Part model, mm, in its own coordinate system. Face numbers are marked on the shaded views. A direction names the side the tool comes from. Round coordinates to 2 decimals unless told otherwise and drop trailing zeros. Loops run counter-clockwise (first coordinate to the right, second up) from the corner with the lowest first, then second, coordinate; pieces in that order, holes last. Notation, with made-up numbers: (-32.5, 52.5) -> (-10.5, 52.5) arc R5 cw to (-10.5, 57.5) -> close; hole circle Ø10 at (9.5, -36.5). An arc over 180 degrees is marked (long way). Answer as CSV lines item,"result".
Autodesk Inventor part; units mm, degrees
ref_plane "YZ Plane" through (0, 0, 0) normal (1, 0, 0) x (0, 1, 0)
ref_plane "XZ Plane" through (0, 0, 0) normal (0, 1, 0) x (-1, 0, 0)
ref_plane "XY Plane" through (0, 0, 0) normal (0, 0, 1) x (1, 0, 0)
sketch "Sketch1" plane through (0, 0, 0) normal (0, 1, 0) x (-1, 0, 0)
  circle A0 centre (0, 0) radius 4.953
  circle A1 centre (0, -11.43) radius 4.953
  dimension "d0" = 9.906
  dimension "d1" = 9.906
  dimension "d2" = 11.43
extrude "Extrusion1" add sketch "Sketch1" along normal blind 1.2192
sketch "Sketch2" plane through (0, 1.2192, 0) normal (0, 1, 0) x (1, 0, 0)
  circle A0 centre (0, 0) radius 3.683
  circle A1 centre (0, 11.43) radius 3.683
  dimension "d5" = 7.366
  dimension "d6" = 7.366
  dimension "d7" = 11.43
extrude "Extrusion2" add sketch "Sketch2" along normal blind 6.731
fillet "Fillet1" radius 0.7937 2 edges at (-3.683, 7.9502, -11.43) (-3.683, 7.9502, 0)
sketch "Sketch3" plane through (0, 0, 0) normal (0, -1, 0) x (1, 0, 0)
  circle A0 centre (0, 0) radius 2.8892
  line L0 (-4.953, 0) -> (-6.0325, 0)
  line L1 (-7.62, -1.5875) -> (-7.62, -9.8425)
  line L2 (-4.953, -11.43) -> (-6.0325, -11.43)
  circle A1 centre (0, -11.43) radius 4.953
  line L3 (4.953, -11.4315) -> (6.039, -11.4309)
  line L4 (7.6256, -9.8425) -> (7.6209, -1.5873)
  line L5 (6.0334, -0.0007) -> (4.953, -0.0007)
  line L6 (-6.35, -8.5725) -> (-6.35, -2.8575)
  line L7 (-4.7625, -1.27) -> (-4.7874, -1.27)
  line L8 (-4.7874, -10.16) -> (-4.7625, -10.16)
  circle A2 centre (0, 0) radius 4.953
  line L9 (4.7874, -1.27) -> (4.7641, -1.27)
  line L10 (6.3516, -2.8566) -> (6.3548, -8.5716)
  line L11 (4.7682, -10.16) -> (4.7874, -10.16)
  arc A3 (6.039, -11.4309) -> (7.6256, -9.8425) centre (6.0381, -9.8434) ccw
  arc A4 (4.7682, -10.16) -> (6.3548, -8.5716) centre (4.7673, -8.5725) ccw
  arc A5 (7.6209, -1.5873) -> (6.0334, -0.0007) centre (6.0334, -1.5882) ccw
  arc A6 (6.3516, -2.8566) -> (4.7641, -1.27) centre (4.7641, -2.8575) ccw
  arc A7 (-6.0325, 0) -> (-7.62, -1.5875) centre (-6.0325, -1.5875) ccw
  arc A8 (-4.7625, -1.27) -> (-6.35, -2.8575) centre (-4.7625, -2.8575) ccw
  arc A9 (-6.35, -8.5725) -> (-4.7625, -10.16) centre (-4.7625, -8.5725) ccw
  arc A10 (-7.62, -9.8425) -> (-6.0325, -11.43) centre (-6.0325, -9.8425) ccw
  circle A11 centre (0, -11.43) radius 2.8892
  point P0 (7.6265, -11.43)
  dimension "d12" = 1.27
  dimension "d14" = 1.5875
  dimension "d17" = 7.62
  dimension "d18" = 1.27
  dimension "d21" = 7.62
  dimension "d22" = 1.27
  dimension "d23" = 1.2716
extrude "Extrusion3" add sketch "Sketch3" against normal blind 1.2192 contours A2 A8 L6 A9 A1 L2 A10 L1 A7 L0 | L5 A5 L4 A3 L3 A1 A4 L10 A6 A2
properties part number "push_buttons"
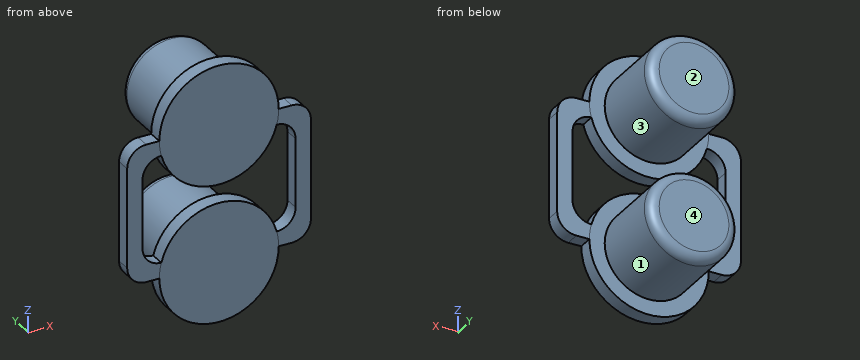
Q1. Saw through at D-D, the plane y = 5.75. Write the cut outline in (x, z), then the cut area to 3 significant figures.
Geometry results:
outline,"circle Ø7.37 at (0, -11.43); circle Ø7.37 at (0, 0)"
area,"85.2 mm2"
Q2. Saw through at B-B, the plane z = -6.75. Write the cut outline in (x, y), then the cut area to 3 significant figures.
Geometry results:
outline,"(-7.62, 0) -> (-6.35, 0) -> (-6.35, 1.22) -> (-7.62, 1.22) -> close; (-1.62, 0) -> (1.62, 0) -> (1.62, 1.22) -> (-1.62, 1.22) -> close; (6.35, 0) -> (7.62, 0) -> (7.62, 1.22) -> (6.35, 1.22) -> close"
area,"7.05 mm2"
Q3. Drill centre lines: line 1 along Z through (x, y) = (0, 6); line 2 along Z through (x, y) = (2, 0.5); line 3 along Y through (x, z) = (2, 4.25). Where is each one in solid material? Low to high.
Geometry results:
line 1,"-15.11 to -7.75, -3.68 to 3.68"
line 2,"-15.96 to -6.9, -4.53 to 4.53"
line 3,"0 to 1.22"
Q4. Saw through at A-A, the plane x = 0. Write the cut outline in (y, z), then the cut area to 3 significant figures.
Geometry results:
outline,"(0, -16.38) -> (1.22, -16.38) -> (1.22, -15.11) -> (7.16, -15.11) arc R0.79 ccw to (7.95, -14.32) -> (7.95, -8.54) arc R0.79 ccw to (7.16, -7.75) -> (1.22, -7.75) -> (1.22, -6.48) -> (0, -6.48) -> close; (0, -4.95) -> (1.22, -4.95) -> (1.22, -3.68) -> (7.16, -3.68) arc R0.79 ccw to (7.95, -2.89) -> (7.95, 2.89) arc R0.79 ccw to (7.16, 3.68) -> (1.22, 3.68) -> (1.22, 4.95) -> (0, 4.95) -> close"
area,"123 mm2"
Q5. Which spindle directions (+Z, -Z, +X, -X, +Y, -Y) get a long thin tool onto all of the face, cutting with end or side? Do the marked faces 3 and 4. Say none if no direction does.
Geometry results:
face 3,"+Y"
face 4,"+Z, -Z, +X, -X, +Y"
Q6. Drop flat-ended pins along their axis: P1, Ø0.5, axis at x = 5.5, y = 0.5, coming from the +Z side; P2, Ø1.5, axis at x = 4, y = 3, coming from the -Z side; P3, Ø2, axis at y = 3, z = -6.5, coming from the +X side; P4, Ø1, axis at x = -2.5, y = 7, coming from the +Z side. Give the stop position or say it passes through.
Geometry results:
P1,"z = 0"
P2,"z = -13.16"
P3,"through"
P4,"z = 3.09"
Q7. Two-plate mould, pull along Z, no slides. Class the marked faces 1 and 2: pulls with the +Z half, pulls with the -Z half, needs draft (parallel to the pull), parting line crosses it, or undercut.
Geometry results:
face 1,"undercut"
face 2,"needs draft"
